Autodesk Inventor part; units mm, degrees
ref_plane "YZ Plane" through (0, 0, 0) normal (1, 0, 0) x (0, 1, 0)
ref_plane "XZ Plane" through (0, 0, 0) normal (0, 1, 0) x (-1, 0, 0)
ref_plane "XY Plane" through (0, 0, 0) normal (0, 0, 1) x (1, 0, 0)
sketch "Эскиз8" plane through (0, 0, 0) normal (1, 0, 0) x (0, 1, 0)
  line L0 (0, 0) -> (10.4, 0)
  line L1 (10.4, 0) -> (10.4, -10.4)
  line L2 (10.4, -10.4) -> (0, -10.4)
  line L3 (0, -10.4) -> (0, 0)
  line L4 (5.2, 0) -> (5.2, 4)
  line L5 (5.2, -10.4) -> (5.2, -14.4)
  circle A0 centre (5.2, 4) radius 1.6
  circle A1 centre (5.2, -14.4) radius 1.6
  line L6 (5.2, 4) -> (7.9, 4)
  line L7 (7.9, 2.4412) -> (5.2, 0.8823)
  line L8 (5.2, 0.8823) -> (2.5, 2.4412)
  line L9 (2.5, 2.4412) -> (2.5, 5.5588)
  line L10 (2.5, 5.5588) -> (5.2, 7.1177)
  line L11 (5.2, 7.1177) -> (7.9, 5.5588)
  line L12 (7.9, 5.5588) -> (7.9, 2.4412)
  line L13 (7.9, -15.9588) -> (5.2, -17.5177)
  line L14 (5.2, -17.5177) -> (2.5, -15.9588)
  line L15 (2.5, -15.9588) -> (2.5, -12.8412)
  line L16 (2.5, -12.8412) -> (5.2, -11.2823)
  line L17 (5.2, -11.2823) -> (7.9, -12.8412)
  line L18 (7.9, -12.8412) -> (7.9, -15.9588)
  circle A2 centre (5.2, 4) radius 5.2
  circle A3 centre (5.2, -14.4) radius 5.2
  line L19 (10.4, 4) -> (10.4, 0)
  line L20 (10.4, -10.4) -> (10.4, -14.4)
  line L21 (0, -14.4) -> (0, -10.4)
  line L22 (0, 4) -> (0, 0)
  line L23 (7.9, 5.5588) -> (7.9, 8.4441)
  line L24 (2.5, 5.5588) -> (2.5, 8.4441)
  line L25 (2.5, -15.9588) -> (2.5, -18.8441)
  line L26 (7.9, -15.9588) -> (7.9, -18.8441)
  line L27 (0, 0) -> (-3, 0)
  line L28 (-3, 0) -> (-3, -10.4)
  line L29 (-3, -10.4) -> (0, -10.4)
  line L30 (0, -10.4) -> (0, 0)
  line L31 (10.4, 0) -> (8.9, 2.5981)
  line L32 (10.4, -10.4) -> (8.9, -12.9981)
  line L33 (10.4, -10.4) -> (13.4, -10.4) construction
  line L34 (8.9, -12.9981) -> (4.4, -10.4)
  line L35 (8.9, 2.5981) -> (4.4, 0)
  line L36 (-3, 0) -> (0.663, 6.5408)
  line L37 (-3, -10.4) -> (0.663, -16.9408)
  line L38 (10.4, 0) -> (12.9981, 1.5)
  line L39 (12.9981, 1.5) -> (9.5707, 6.8173)
  line L40 (10.4, -10.4) -> (12.9981, -11.9)
  line L41 (12.9981, -11.9) -> (9.5707, -17.2173)
  point P0 (7.9, -14.4)
  dimension "d51" = 10.4
  dimension "d52" = 10.4
  dimension "d53" = 4
  dimension "d54" = 4
  dimension "d55" = 3.2
  dimension "d56" = 3.2
  dimension "d57" = 2.7
  dimension "d58" = 3
  dimension "d59" = 3
  dimension "d60" = 3
  dimension "d61" = 120
  dimension "d62" = 3
  dimension "d63" = 3
extrude "Выдавливание6" add sketch "Эскиз8" along normal blind 5 contours L0 A2 L24 L9 L8 L4 L35 | L0 L22 A2 | L4 L7 L12 L23 A2 L31 L35 | L27 L36 A2 L22 | L3 L29 L28 L27 | L31 A2 L19 | L19 A2 L39 L38 | L2 A3 L21 | L21 A3 L37 L29 | L40 L41 A3 L20 | L20 A3 L32 | L2 L34 L5 L16 L15 L25 A3 | A3 L26 L18 L17 L5 L34 L32
sketch "Эскиз9" plane through (0, 0, 0) normal (-1, 0, 0) x (0, 0, 1)
  arc A0 (-18.8441, 2.5) -> (-16.9408, 0.663) centre (-14.4, 5.2) ccw
  circle A1 centre (-14.4, 5.2) radius 5.2
  circle A2 centre (-14.4, 5.2) radius 1.6
  arc A3 (6.5408, 0.663) -> (8.4441, 2.5) centre (4, 5.2) ccw
  circle A4 centre (4, 5.2) radius 5.2
  circle A5 centre (4, 5.2) radius 1.6
  line L0 (2.5981, 8.9) -> (0, 10.4)
  line L1 (0, 10.4) -> (2.5981, 8.9)
  line L2 (0, 4.4) -> (2.5981, 8.9)
  line L3 (2.5981, 8.9) -> (0, 4.4)
  line L4 (0, 0) -> (0, 4.4)
  line L5 (0, 4.4) -> (0, 0)
  line L6 (-10.4, 4.4) -> (-10.4, 0)
  line L7 (0, 0) -> (-10.4, 0)
  line L8 (-10.4, 0) -> (-10.4, 1.8774)
  line L9 (-10.4, 10.4) -> (-12.9981, 8.9)
  line L10 (-11.699, 9.65) -> (-10.4, 10.4)
  line L11 (-11.9, 12.9981) -> (-10.4, 10.4)
  line L12 (-10.4, 10.4) -> (-11.9, 12.9981)
  line L13 (-17.2173, 9.5707) -> (-11.9, 12.9981)
  line L14 (-11.9, 12.9981) -> (-17.2173, 9.5707)
  line L15 (0, 10.4) -> (1.5, 12.9981)
  line L16 (0, 10.4) -> (1.5, 12.9981)
  line L17 (1.5, 12.9981) -> (6.8173, 9.5707)
  line L18 (1.5, 12.9981) -> (6.8173, 9.5707)
  line L19 (0, -3) -> (-10.4, -3)
  line L20 (0, -3) -> (6.5408, 0.663)
  line L21 (6.5408, 0.663) -> (0, -3)
  line L22 (-10.4, -3) -> (-16.9408, 0.663)
  line L23 (-10.4, -3) -> (-16.9408, 0.663)
  line L24 (-10.4, -3) -> (0, -3)
  line L25 (-10.4, 0) -> (0, 0)
  line L26 (0, 0) -> (-10.4, 0)
  line L27 (-10.4, 0) -> (-10.4, 1.8774)
  line L28 (0, 1.8774) -> (0, 0)
  line L29 (-11.699, 9.65) -> (-12.9981, 8.9)
  line L30 (-12.9981, 8.9) -> (-10.4, 4.4)
  line L31 (-10.4, 4.4) -> (-12.9981, 8.9)
  line L32 (-12.9981, 8.9) -> (-10.4, 4.4)
  line L33 (-10.4, 4.4) -> (-10.4, 1.8774)
  line L34 (0, 1.8774) -> (0, 4.4)
  line L35 (2.5981, 8.9) -> (0, 4.4)
  line L36 (1.299, 9.65) -> (2.5981, 8.9)
  point P0 (-18.8441, 2.5)
  point P1 (-16.9408, 0.663)
  point P2 (6.5408, 0.663)
  point P3 (8.4441, 2.5)
  dimension "d66" = 3.2
  dimension "d67" = 3.2
extrude "Выдавливание7" add sketch "Эскиз9" along normal blind 5 contours A1 L9 L30 L6 A0 | A1 L6 L7 L4 A4 L20 L19 L22 | L13 L11 L9 A1 | A4 L4 L2 L0 A3 | L0 L15 L17 A4
sketch "Эскиз10" plane through (5, 0, 0) normal (1, 0, 0) x (0, 0, -1)
  line L0 (-1.5, 12.9981) -> (-6.8173, 9.5707)
  line L1 (0, 10.4) -> (-1.5, 12.9981)
  line L2 (-1.5, 12.9981) -> (0, 10.4)
  line L3 (-2.5981, 8.9) -> (0, 10.4)
  line L4 (0, 10.4) -> (-2.5981, 8.9)
  line L5 (0, 4.4) -> (-2.5981, 8.9)
  line L6 (-2.5981, 8.9) -> (0, 4.4)
  line L7 (0, 0) -> (0, 4.4)
  line L8 (0, 4.4) -> (0, 0)
  line L9 (10.4, 0) -> (0, 0)
  line L10 (0, 0) -> (10.4, 0)
  line L11 (10.4, 4.4) -> (10.4, 0)
  line L12 (10.4, 0) -> (10.4, 4.4)
  line L13 (10.4, 10.4) -> (12.9981, 8.9)
  line L14 (10.4, 4.4) -> (12.9981, 8.9)
  line L15 (12.9981, 8.9) -> (10.4, 10.4)
  line L16 (11.9, 12.9981) -> (10.4, 10.4)
  line L17 (10.4, 10.4) -> (11.9, 12.9981)
  line L18 (17.2173, 9.5707) -> (11.9, 12.9981)
  line L19 (11.9, 12.9981) -> (17.2173, 9.5707)
  line L20 (17.2173, 9.5707) -> (13.6704, -1.1685)
  line L21 (10.4, -3) -> (16.9408, 0.663)
  line L22 (10.4, -3) -> (13.6704, -1.1685)
  line L23 (0, -3) -> (10.4, -3)
  line L24 (-6.5408, 0.663) -> (0, -3)
  line L25 (10.4, -3) -> (0, -3)
  arc A0 (-8.4441, 2.5) -> (-6.5408, 0.663) centre (-4, 5.2) ccw
  line L26 (0, -3) -> (-6.5408, 0.663)
  line L27 (-3.2704, -1.1685) -> (-6.8173, 9.5707)
  line L28 (-6.8173, 9.5707) -> (-1.5, 12.9981)
extrude "Выдавливание8" add sketch "Эскиз10" along normal blind 157.53
sketch "Эскиз17" plane through (-5, 0, 0) normal (-1, 0, 0) x (0, 0, 1)
  line L0 (-37.7292, 41.1824) -> (41.3103, 41.1824)
  line L1 (41.3103, 41.1824) -> (41.3103, -34.7876)
  line L2 (41.3103, -34.7876) -> (-37.7292, -34.7876)
  line L3 (-37.7292, -34.7876) -> (-37.7292, 41.1824)
  point P0 (0, 0)
extrude "Выдавливание13" cut sketch "Эскиз17" against normal blind 147.53
sketch "Эскиз23" plane through (162.53, 0, 0) normal (1, 0, 0) x (0, 0, -1)
  point P0 (0, 0)
fillet "Сопряжение12" radius 4 6 edges at (152.53, -3, -10.4) (152.53, -1.1685, -13.6704) (152.53, -3, 0) (152.53, -1.1685, 3.2704) (152.53, 9.5707, -17.2173) (152.53, 9.5707, 6.8173)
sketch "Эскиз24" plane through (142.53, 0, 0) normal (-1, 0, 0) x (0, 0, 1)
  line L0 (-11.9, 12.9981) -> (-10.4, 10.4)
  line L1 (-11.9, 12.9981) -> (1.5, 12.9981)
  line L2 (1.5, 12.9981) -> (1.5, 16.9981)
  line L3 (1.5, 16.9981) -> (-11.9, 16.9981)
  line L4 (-11.9, 16.9981) -> (-11.9, 12.9981)
  line L5 (1.5, 16.9981) -> (-11.9, 16.9981)
  line L6 (-11.9, 16.9981) -> (-11.9, 19.9981)
  line L7 (-11.9, 19.9981) -> (1.5, 19.9981)
  line L8 (1.5, 19.9981) -> (1.5, 16.9981)
  line L9 (-11.9, 16.9981) -> (-11.7, 16.9981) construction
  line L10 (-14.6154, 11.2478) -> (-11.9, 12.9981)
  line L11 (-12.1, 12.9981) -> (-11.9, 12.9981)
  line L12 (1.5, 12.9981) -> (1.7, 12.9981)
  line L13 (1.7, 13.7481) -> (1.7, 19.9981)
  line L14 (1.7, 19.9981) -> (1.5, 19.9981)
  line L15 (-12.1, 13.7481) -> (-12.1, 19.9981)
  line L16 (-12.1, 19.9981) -> (-11.9, 19.9981)
  line L17 (-12.1, 16.9981) -> (-11.9, 16.9981)
  line L18 (1.5, 16.9981) -> (1.7, 16.9981)
  line L19 (-12.85, 12.9981) -> (-12.85, 12.9981)
  line L20 (-13.6, 13.7481) -> (-13.6, 28.4571)
  line L21 (-13.6, 29.9981) -> (-12.1, 29.9981)
  line L22 (-12.1, 29.9981) -> (-12.1, 12.9981)
  line L23 (2.45, 12.9981) -> (2.45, 12.9981)
  line L24 (3.2, 13.7481) -> (3.2, 28.4571)
  line L25 (3.2, 29.9981) -> (1.7, 29.9981)
  line L26 (1.7, 29.9981) -> (1.7, 12.9981)
  line L27 (-13.7992, 28.47) -> (-16.4147, 8.4027)
  arc A0 (-14.6154, 11.2478) -> (-16.2465, 6.6313) centre (-12.4482, 7.8857) ccw
  line L28 (3.3992, 28.47) -> (6.0147, 8.4027)
  arc A1 (5.8465, 6.6313) -> (4.2154, 11.2478) centre (2.0482, 7.8857) ccw
  arc A2 (-12.85, 12.9981) -> (-12.1, 13.7481) centre (-12.85, 13.7481) ccw
  arc A3 (-13.6, 13.7481) -> (-12.85, 12.9981) centre (-12.85, 13.7481) ccw
  arc A4 (1.7, 13.7481) -> (2.45, 12.9981) centre (2.45, 13.7481) ccw
  arc A5 (2.45, 12.9981) -> (3.2, 13.7481) centre (2.45, 13.7481) ccw
  line L29 (-14.1579, 0.3075) -> (-16.2465, 6.6313)
  line L30 (-16.2465, 6.6313) -> (-14.1579, 0.3075)
  circle A6 centre (-12.4482, 7.8857) radius 4
  line L31 (5.8465, 6.6313) -> (3.7579, 0.3075)
  circle A7 centre (2.0482, 7.8857) radius 4
  arc A8 (1.9142, -1.928) -> (3.7579, 0.3075) centre (-0.0403, 1.562) ccw
  circle A9 centre (-0.0403, 1.562) radius 4
  arc A10 (-1.0438, -3) -> (0.9107, -2.49) centre (-1.0438, 1) ccw
  circle A11 centre (-1.0438, 1) radius 4
  line L32 (-10.4, 4.4) -> (-10.4, 0)
  circle A12 centre (-10.4, 1.562) radius 4.0051
  arc A13 (-11.3107, -2.49) -> (-9.3562, -3) centre (-9.3562, 1) ccw
  circle A14 centre (-9.3562, 1) radius 4
  arc A15 (-14.1579, 0.3075) -> (-12.3142, -1.928) centre (-10.3597, 1.562) ccw
  line L33 (-12.3142, -1.928) -> (-11.3107, -2.49)
  line L34 (1.9142, -1.928) -> (0.9107, -2.49)
  line L35 (1.9142, -1.928) -> (0.9107, -2.49)
  line L36 (-1.0438, -3) -> (-9.3562, -3)
  line L37 (-9.3562, -3) -> (-1.0438, -3)
  line L38 (0.9107, -2.49) -> (-0.2774, -3.1554)
  line L39 (-11.3107, -2.49) -> (-10.1226, -3.1554)
  line L40 (2.0482, 7.8857) -> (6.0482, 7.8857)
  line L41 (6.0482, 7.8857) -> (9.0482, 7.8857)
  line L42 (-16.4482, 7.8857) -> (-19.4482, 7.8857)
  line L43 (-19.4482, 7.8857) -> (-14.9537, -3.9206)
  line L44 (-13.6, 29.9981) -> (-13.6, 31.9981)
  line L45 (3.2, 29.9981) -> (3.2, 31.9981)
  arc A16 (3.2, 31.9981) -> (1.7, 29.9981) centre (3.699, 30.0613) ccw
  arc A17 (-12.1, 29.9981) -> (-13.6, 31.9981) centre (-14.099, 30.0613) ccw
  arc A18 (3.3992, 28.47) -> (3.2, 28.4571) centre (3.3, 28.4571) ccw
  arc A19 (-13.6, 28.4571) -> (-13.7992, 28.47) centre (-13.7, 28.4571) ccw
  line L46 (3.2, 31.9981) -> (4.2, 31.9976)
  line L47 (4.2, 31.9976) -> (9.0482, 7.8857)
  line L48 (-13.6, 31.9981) -> (-14.6, 31.9981)
  line L49 (-14.6, 31.9981) -> (-19.4482, 7.8857)
  line L50 (9.0482, 7.8857) -> (4.5537, -3.9206)
  circle A20 centre (0.1512, -3.9206) radius 0.8771
  circle A21 centre (-10.5512, -3.9206) radius 0.8771
  line L51 (4.5537, -3.9206) -> (9.0482, -6.5155)
  line L52 (4.5537, -3.9206) -> (9.7436, -3.9206) construction
  line L53 (9.0482, -6.5155) -> (-0.0136, -4.7821)
  line L54 (-14.9537, -3.9206) -> (-19.4482, -6.5155)
  line L55 (-14.9537, -3.9206) -> (-9.7638, -3.9206) construction
  line L56 (-19.4482, -6.5155) -> (-10.3864, -4.7821)
  point P0 (0, 0)
  point P1 (-13.6, 12.9981)
  point P2 (3.2, 12.9981)
  point P3 (-15.1183, -5.3024)
  point P4 (-11.3107, -2.49)
  point P5 (-11.9564, -2.1284)
  point P6 (-14.3463, 0.8779)
  dimension "d145" = 4
  dimension "d149" = 0.2
  dimension "d150" = 1.5
  dimension "d151" = 17
  dimension "d152" = 1.5
  dimension "d153" = 17
  dimension "d154" = 0.75
  dimension "d161" = 3
  dimension "d162" = 3
  dimension "d163" = 2
  dimension "d164" = 2
  dimension "d165" = 2
  dimension "d166" = 0.1
  dimension "d167" = 1
  dimension "d168" = 1
  dimension "d187" = 30
  dimension "d188" = 150
extrude "Выдавливание17" add sketch "Эскиз24" along normal blind 10 contours L6 L7 L8 L3 | L17 L15 L16 L6 | L8 L14 L13 L18 | L15 A2 A3 L20 A19 L27 A0 L42 L49 L48 L44 L21 L22 | L13 L26 L25 L45 L46 L47 L41 A1 L28 A18 L24 A5 A4 | A0 L29 A12 L33 L39 A21 L56 L54 L43 L42 | L21 L44 A17 | A16 L45 L25 | A21 | L34 A8 L31 A1 L41 L50 L51 L53 A20 L38 | A20
fillet "Сопряжение13" radius 0.3 4 edges at (137.53, 31.9976, 4.2) (137.53, 31.9981, -14.6) (137.53, -6.5155, 9.0482) (137.53, -6.5155, -19.4482)
sketch "Эскиз25" plane through (162.53, 0, 0) normal (1, 0, 0) x (0, 0, -1)
  line L0 (-19.4307, 22.3831) -> (30.691, 22.3831)
  line L1 (30.691, 22.3831) -> (30.691, -15.6545)
  line L2 (30.691, -15.6545) -> (-19.4307, -15.6545)
  line L3 (-19.4307, -15.6545) -> (-19.4307, 22.3831)
  point P0 (0, 0)
extrude "Выдавливание18" cut sketch "Эскиз25" against normal blind 20
sketch "Эскиз28" plane through (132.53, 19.9981, -12.1) normal (0, 1, 0) x (1, 0, 0)
  line L0 (0, -13.8) -> (0, 0)
  line L1 (0, -6.9) -> (10, -6.9)
  line L2 (10, -13.8) -> (10, 0)
  circle A0 centre (5, -6.9) radius 1.6
  point P0 (-132.53, -12.1)
  dimension "d189" = 3.2
extrude "Выдавливание21" cut sketch "Эскиз28" against normal blind 10
sketch "Эскиз29" plane through (132.53, 19.9981, -12.1) normal (0, 1, 0) x (1, 0, 0)
  circle A0 centre (5, -6.9) radius 1.6
  line L0 (5, -6.9) -> (7.7, -6.9)
  line L1 (7.7, -8.4588) -> (5, -10.0177)
  line L2 (5, -10.0177) -> (2.3, -8.4588)
  line L3 (2.3, -8.4588) -> (2.3, -5.3412)
  line L4 (2.3, -5.3412) -> (5, -3.7823)
  line L5 (5, -3.7823) -> (7.7, -5.3412)
  line L6 (7.7, -5.3412) -> (7.7, -8.4588)
  point P0 (-132.53, -12.1)
  dimension "d192" = 2.7
extrude "Выдавливание22" cut sketch "Эскиз29" against normal blind 1.5
properties part number "защёлка_выдача2"
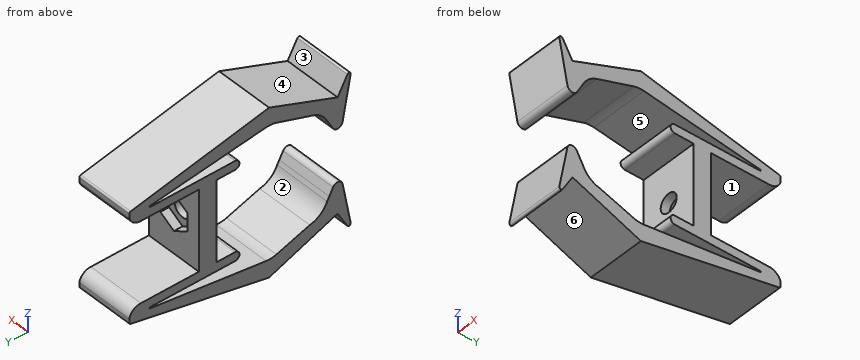
Check sheet for the modelled part. Datum: model origin and axes. Units: mm. Face numbers are marked on the shaded views. A direction names the side the tool comes from. Give positions to 0.01 mm unless a question says otherwise; leave off trailing zeros. Write each loop counter-clockwise with the first axis right and the second up, starting at its lowest first coordinate (ties: lowest second). Pieces come first, ordered by that corner, then holes.
Item 1: Gauge pin test, flat ends, axial feed: pin 1 (1 mm diameter, centred on x = 137.5, y = 15, fed in from +Z); pin 2 (4.5 mm diameter, centred on x = 137, z = -4, fed in from +Y); pin 3 (1.5 mm diameter, centred on x = 134.5, y = 24, fed in from -Z). Record the tip position at first contact, or that the pin passes through.
Item 2: Cross-section at D-D (z = -12.85). Enter the section's corners in (x, y), and give its area (3 significant figures).
Item 3: Cross-section at B-B (y = 27). Enter the section's corners in (x, z).
Item 4: Scan lines: L1, parallel to X at y = 18.1, z = -5.2; L2, parallel to Z at x = 135.75, y = 25; L3, parallel to Z at x = 137.53, y = 17.7. Record each from-to range of solid material in increasing order.
Item 5: Draft check along Z on the marked faces 4, 5 and 6. Enter one of: released by +Z, released by -Z, zero draft, split by the parting line, or undercut.
Item 6: Cross-section at A-A (z = -5.2). Enter the section's corners in (x, y).
Item 7: Cross-section at C-C (y = -0.5). Enter the section's corners in (x, z).
Item 8: Access from +Z, -Z, +X, -X, +Y, -Y to the whole of each face (thin tool, end or side, straight path). Record for the marked faces 1, 2 and 3.
Report:
1. pin 1: stops at z = 7.72
1. pin 2: stops at y = 20
1. pin 3: stops at z = -16.36
2. outline: (132.53, -5.25) - (142.53, -5.25) - (142.53, -1.61) - (132.53, -1.61) - close; (132.53, 13) - (142.53, 13) - (142.53, 31.62) - (132.53, 31.62) - close
2. area: 223 mm2
3. outline: (132.53, -15.6) - (142.53, -15.6) - (142.53, -13.99) - (132.53, -13.99) - close; (132.53, -13.6) - (142.53, -13.6) - (142.53, -12.1) - (132.53, -12.1) - close; (132.53, 1.7) - (142.53, 1.7) - (142.53, 3.2) - (132.53, 3.2) - close; (132.53, 3.59) - (142.53, 3.59) - (142.53, 5.2) - (132.53, 5.2) - close
4. L1: x = 132.53 to 135.93, 139.13 to 142.53
4. L2: z = -16.01 to -14.25, -13.6 to -12.1, 1.7 to 3.2, 3.85 to 5.61
4. L3: z = -17.47 to -15.2, -13.6 to -6.8, -3.6 to 3.2, 4.8 to 7.07
5. face 4: released by +Z
5. face 5: undercut
5. face 6: released by -Z
6. outline: (132.53, 17) - (135.93, 17) - (135.93, 18.5) - (134.83, 18.5) - (134.83, 20) - (132.53, 20) - close; (139.13, 17) - (142.53, 17) - (142.53, 20) - (140.23, 20) - (140.23, 18.5) - (139.13, 18.5) - close
7. outline: (132.53, -16.26) - (142.53, -16.26) - (142.53, -13.83) - (132.53, -13.83) - close; (132.53, 3.39) - (142.53, 3.39) - (142.53, 5.86) - (132.53, 5.86) - close
8. face 1: +X, -X, +Y
8. face 2: +X, -X
8. face 3: +Z, +X, -X
